from build123d import *

# Parameters (mm, degrees)
F0_W           = 27
F0_H           = 25
F0_R           = 2
F0_R_2         = 6.5
F1_DEPTH       = 12
F2_W           = 2
F2_H           = 25
F3_DEPTH       = 28
F4_R           = 1.5
F5_DEPTH       = 4
F6_R           = 1.5
F7_DEPTH       = 4
F8_R           = 1.5
F9_DEPTH       = 4
F10_R          = 3
F11_R          = 3.5
F11_R_2        = 1.5
F12_DEPTH      = 25
F12_DEPTH_BACK = 25


with BuildPart() as f1:
    # F0 (on Top) → F1 (new body)
    with BuildSketch(Plane.XY):
        with Locations((0.431113, -5.095445)):
            Rectangle(F0_W, F0_H)
        with Locations((-7.068887, -13.595445)):
            Circle(F0_R, mode=Mode.SUBTRACT)
        with Locations((9.931113, -13.595445)):
            Circle(F0_R, mode=Mode.SUBTRACT)
        with Locations((-7.068887, 3.404555)):
            Circle(F0_R, mode=Mode.SUBTRACT)
        with Locations((3.931113, -5.095445)):
            Circle(F0_R_2, mode=Mode.SUBTRACT)
        with Locations((9.931113, 3.404555)):
            Circle(F0_R, mode=Mode.SUBTRACT)
    extrude(amount=F1_DEPTH)

    # F2 (on face) → F3 (join)
    with BuildSketch(Plane.XY.offset(12)):
        with Locations((-12.068887, -5.095445)):
            Rectangle(F2_W, F2_H)
    extrude(amount=F3_DEPTH)

    # F4 (on face) → F5 (cut)
    with BuildSketch(Plane.YZ.offset(13.931113)):
        with Locations((-9.995445, 6)):
            Circle(F4_R)
        with Locations((0.004555, 6)):
            Circle(F4_R)
    extrude(amount=-F5_DEPTH, mode=Mode.SUBTRACT)

    # F6 (on face) → F7 (cut)
    with BuildSketch(Plane.XZ.offset(17.595445)):
        with Locations((-1.068887, 6)):
            Circle(F6_R)
    extrude(amount=-F7_DEPTH, mode=Mode.SUBTRACT)

    # F8 (on face) → F9 (cut)
    with BuildSketch(Plane(origin=(0, 7.404555, 0), x_dir=(-1, 0, 0), z_dir=(0, 1, 0))):
        with Locations((1.068887, 6)):
            Circle(F8_R)
    extrude(amount=-F9_DEPTH, mode=Mode.SUBTRACT)

    # F10
    f10_edges = [f1.edges().sort_by_distance(p)[0] for p in [
        (13.931113, -17.595445, 6),
        (13.931113, 7.404555, 6),
    ]]
    fillet(f10_edges, radius=F10_R)

    # F11 (on face) → F12 (cut, two sides)
    with BuildSketch(Plane.YZ.offset(-11.068887)) as f12_sk:
        with Locations((-5.095445, 25)):
            Circle(F11_R)
        with Locations((-5.095445, 33.5)):
            Circle(F11_R_2)
        with Locations((-5.095445, 16.5)):
            Circle(F11_R_2)
    extrude(amount=-F12_DEPTH, mode=Mode.SUBTRACT)
    extrude(f12_sk.sketch, amount=-F12_DEPTH_BACK, mode=Mode.SUBTRACT)


solid = f1.part
Input: part model. Units: mm. Frame: model coordinates. A direction names the side the tool comes from. Coordinates: 2 decimals unless noted, no trailing zeros. Loops run counter-clockwise (first coordinate to the right, second up) from the corner with the lowest first, then second, coordinate; pieces in that order, holes last. Notation, with made-up numbers: (78.25, 8.5) -> (85.25, 8.5) arc R22 ccw to (85.25, 29.5) -> close; hole circle Ø5 at (-34, -16). An arc over 180 degrees is marked (long way). One line per item, written item: value.
(1) Cut plane C-C (y = -10). Output: boundary loops of the cut face in (x, z), then the cut area to 3 significant figures.
Answer below:
outline: (-13.07, 0) -> (-0.33, 0) -> (-0.33, 12) -> (-11.07, 12) -> (-11.07, 40) -> (-13.07, 40) -> close; (8.2, 0) -> (13.93, 0) -> (13.93, 4.5) -> (9.93, 4.5) -> (9.93, 7.5) -> (13.93, 7.5) -> (13.93, 12) -> (8.2, 12) -> close
area: 266 mm2
(2) Set-up query: faces 1 (the face through (-1, 3.405, 6)), 2 (the face through (9.931, 0, 6)), 3 (the face through (-4, -5, 12)). Return all of +Z, -Z, +X, -X, +Y, -Y with unobstructed straight access to the full face (end or side cutting, diameter ignored); none if empty.
Answer below:
face 1: +Y
face 2: +X
face 3: +Z, +X, +Y, -Y
(3) Pin query (flat end, axial travel): pin 1 Ø1.5 at (y, z) = (-8.5, 18.5) entering from +X; pin 2 Ø1.8 at (y, z) = (0, 6) entering from +X; pin 3 Ø0.9 at (x, z) = (-1, 5.5) entering from -Y. Return the tip coordinate at first contact, or that it passes through.
Answer below:
pin 1: stops at x = -11.07
pin 2: stops at x = 9.93
pin 3: stops at y = -13.6
(4) Ray query, line 1 along X through (y, z) = (3.25, 20); line 2 along Z through (x, y) = (-1, -14.5); line 3 along Z through (x, y) = (-6.75, 1). Return the intervals inside material, ascending.
Answer below:
line 1: x = -13.07 to -11.07
line 2: z = 0 to 4.5, 7.5 to 12
line 3: z = 0 to 12
(5) Draft query along Y for faces 4 (the face through (-11.069, -5, 29)), 5 (the face through (-4, -17.595, 11)), 6 (the face through (-5.161, -12.995, 5.916)), 7 (the face through (11.96, -1.19, 5.09)). Return one class per face: pulls with the +Y half, pulls with the -Y half, needs draft (parallel to the pull), parting line crosses it, or undercut.
Answer below:
face 4: needs draft
face 5: pulls with the -Y half
face 6: undercut
face 7: undercut
(6) Cut plane B-B (x = 2.5). Output: boundary loops of the cut face in (y, z).
Answer below:
outline: (-17.6, 0) -> (-11.44, 0) -> (-11.44, 12) -> (-17.6, 12) -> close; (1.25, 0) -> (7.4, 0) -> (7.4, 12) -> (1.25, 12) -> close
(7) Cut plane D-D (z = 3.5). Output: boundary loops of the cut face in (x, y), then the cut area to 3 significant figures.
Answer below:
outline: (-13.07, -17.6) -> (10.93, -17.6) arc R3 ccw to (13.93, -14.6) -> (13.93, 4.4) arc R3 ccw to (10.93, 7.4) -> (-13.07, 7.4) -> close; hole circle Ø4 at (-7.07, -13.6); hole circle Ø4 at (-7.07, 3.4); hole circle Ø13 at (3.93, -5.1); hole circle Ø4 at (9.93, -13.6); hole circle Ø4 at (9.93, 3.4)
area: 488 mm2
(8) Cut plane A-A (z = 16.5). Output: boundary loops of the cut face in (x, y).
Answer below:
outline: (-13.07, -17.6) -> (-11.07, -17.6) -> (-11.07, -6.6) -> (-13.07, -6.6) -> close; (-13.07, -3.6) -> (-11.07, -3.6) -> (-11.07, 7.4) -> (-13.07, 7.4) -> close
